Design review of the part built by this model. Coordinates are the model's own, in mm. Coordinates: 2 decimals unless noted, no trailing zeros. Order: outer loops, then holes, each group sorted by start corner. A loop starts at its lowest first (then second) coordinate and runs counter-clockwise, first axis right, second up. Notation, with made-up numbers: (24.25, 11) -> (40.25, 11) arc R12 cw to (40.25, 24) -> close; hole circle Ø7 at (24, 38.5). An arc over 180 degrees is marked (long way). Write item = value, one per line.
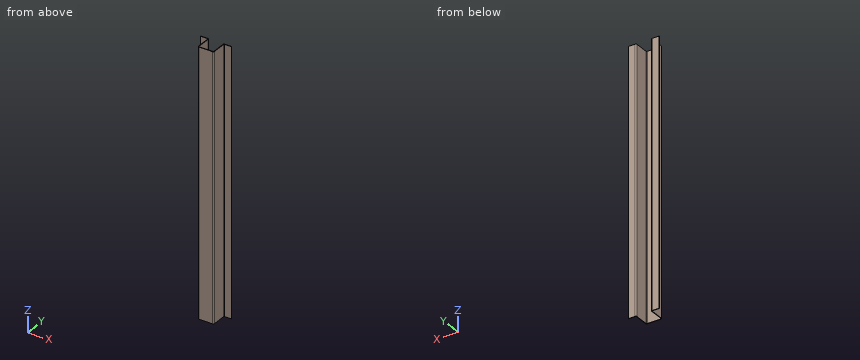
Autodesk Inventor part; units mm, degrees
ref_plane "YZ Plane" through (0, 0, 0) normal (1, 0, 0) x (0, 1, 0)
ref_plane "XZ Plane" through (0, 0, 0) normal (0, 1, 0) x (-1, 0, 0)
ref_plane "XY Plane" through (0, 0, 0) normal (0, 0, 1) x (1, 0, 0)
sketch "Sketch1" plane through (0, 0, 0) normal (0, 1, 0) x (-1, 0, 0)
  line L0 (0, 0) -> (30, 0)
  line L1 (30, 0) -> (30, -496)
  line L2 (30, -496) -> (0, -496)
  line L3 (0, -496) -> (0, 0)
  dimension "d0" = 30
  dimension "d1" = 496
extrude "Plate1" add sketch "Sketch1" along normal blind 1
sketch "Sketch2" plane through (-29, 0, 0) normal (-1, 0, 0) x (0, -1, 0)
  line L0 (0, -496) -> (0, 0)
  line L1 (0, 0) -> (-30, 0)
  line L2 (-30, 0) -> (-30, -496)
  line L3 (-30, -496) -> (0, -496)
edge flange "Flange1" height 30 angle 90 thickness 1 bend radius 1 thickness toward (-1, 0, 0) relief tear relief width 1 relief depth 0.5 corner gap 1 corner form 0 edges at (-30, 1, -248) (0, 1, -248) wall of the first edge with corners at (-29, 0, -496) (-29, 0, 0) (-29, 30, 0) (-29, 30, -496)
bend "Bend1"
corner "Corner1"
sketch "Sketch3" plane through (-29, 29, -496) normal (0, 1, 0) x (-1, 0, 0)
  line L0 (0, 496) -> (0, 0)
  line L1 (0, 0) -> (15, 0)
  line L2 (15, 0) -> (15, 496)
  line L3 (15, 496) -> (0, 496)
edge flange "Flange2" height 15 angle 90 thickness 1 bend radius 1 thickness toward (0, 1, 0) relief tear relief width 1 relief depth 0.5 corner gap 1 corner form 0 edges at (-30, 30, -248) (0, 30, -248) wall of the first edge with corners at (-29, 29, 0) (-29, 29, -496) (-44, 29, -496) (-44, 29, 0)
bend "Bend2"
corner "Corner2"
equation "\"d2\" = Thickness"
equation "\"d3\" = BendReliefWidth"
equation "\"d4\" = BendReliefDepth"
equation "\"d5\" = MinimumRemnant"
equation "\"d6\" = TransitionRadius"
equation "\"d9\" = BendRadius"
equation "\"d10\" = CornerReliefSize"
equation "\"d11\" = GapSize"
equation "\"d12\" = JacobiRadiusSize"
equation "\"d13\" = BendReliefWidth"
equation "\"d14\" = BendReliefDepth"
equation "\"d15\" = MinimumRemnant"
equation "\"d16\" = TransitionRadius"
equation "\"d19\" = BendRadius"
equation "\"d20\" = CornerReliefSize"
equation "\"d21\" = GapSize"
equation "\"d22\" = JacobiRadiusSize"
equation "\"BendRadius\" = Thickness"
equation "\"BendReliefWidth\" = Thickness"
equation "\"BendReliefDepth\" = 0.5 * Thickness"
equation "\"CornerReliefSize\" = 4 * Thickness"
equation "\"MinimumRemnant\" = 2 * Thickness"
equation "\"TransitionRadius\" = BendRadius"
equation "\"JacobiRadiusSize\" = BendRadius"
equation "\"GapSize\" = Thickness"
properties part number "Stringer" material "Aluminum 6061"
(1) We need section A-A (y = 13.25). Write out the cut boundary in (x, z).
Report:
outline = (-30, -496) -> (-29, -496) -> (-29, 0) -> (-30, 0) -> close; (-1, -496) -> (0, -496) -> (0, 0) -> (-1, 0) -> close
(2) We need section B-B (z = -58). Write out the cut boundary in (x, y), and give its area (3 significant figures).
Report:
outline = (-44, 29) -> (-31, 29) arc R1 cw to (-30, 28) -> (-30, 2) arc R2 ccw to (-28, 0) -> (-2, 0) arc R2 ccw to (0, 2) -> (0, 28) arc R1 cw to (1, 29) -> (14, 29) -> (14, 30) -> (1, 30) arc R2 ccw to (-1, 28) -> (-1, 2) arc R1 cw to (-2, 1) -> (-28, 1) arc R1 cw to (-29, 2) -> (-29, 28) arc R2 ccw to (-31, 30) -> (-44, 30) -> close
area = 113 mm²
(3) We need section C-C (x = -16). Write out the cut boundary in (y, z), and give its area (3 significant figures).
Report:
outline = (0, -496) -> (1, -496) -> (1, 0) -> (0, 0) -> close
area = 496 mm²
(4) Insertion check: pin 1 (14.5 mm diameter, centred on x = -39.5, z = -267.5, fed in from -Y); pin 2 (8 mm diameter, centred on y = 15.5, z = -358, fed in from -X); pin 3 (10 mm diameter, centred on x = -9.5, z = -159.5, fed in from +Y); pin 4 (3 mm diameter, centred on x = -27, y = 10, fed in from -Z). Each pin has a flat end and moves straight along its axis. Give the tip position at first contact, or say it passes through.
Report:
pin_1 = 29
pin_2 = -30
pin_3 = 1
pin_4 = through
(5) For L1, parallel to X at y = 4.25, z = -404; L2, parallel to Y at x = -39.5, z = -401; L3, parallel to Y at x = -2, z = -162, list the stretches that pass through material, from the lowest coordinate up.
Report:
L1 = -30 to -29, -1 to 0
L2 = 29 to 30
L3 = 0 to 1
